Verification items for this drawing (mm, ordinates from the low corner). A direction names the side the tool comes from. Give positions to 0.01 mm unless a question says otherwise; leave off trailing zeros. Write each loop counter-clockwise with the first axis right and the second up, starting at its lowest first coordinate (ties: lowest second). Pieces come first, ordered by that corner, then holes. Notation, with made-up numbers: (84, 70.25) -> (97, 70.25) arc R20 cw to (97, 94.25) -> close; hole circle Ø7 at (13, 45). An arc over 180 degrees is marked (long way). Answer as a JSON object with one key per item and string values.
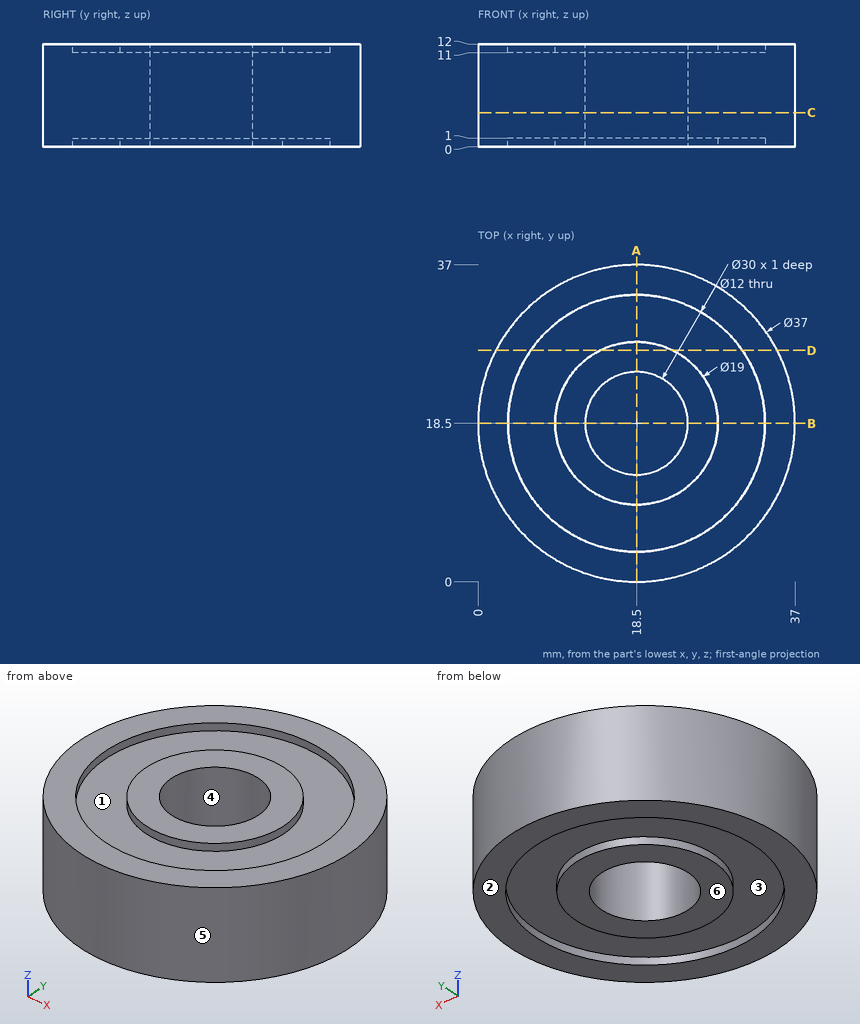
1. Scan lines: L1, parallel to Y at x = 18.5, z = 11.55; L2, parallel to Y at x = 18.5, z = 8; L3, parallel to Z at x = 4.5, y = 21. Record each from-to range of solid material in increasing order. Write a range as [from, to].
Determined:
{"L1": "[0, 3.5], [9, 12.5], [24.5, 28], [33.5, 37]", "L2": "[0, 12.5], [24.5, 37]", "L3": "[1, 11]"}
2. Mould release check, pull along X, two halves, no side actions. Record for the marked faces 4, 5 and 6: released by +X, released by -X, zero draft, split by the parting line, or undercut.
Determined:
{"face 4": "undercut", "face 5": "split by the parting line", "face 6": "zero draft"}
3. Sectioned sample at C-C, the plane z = 4. Enter the section's corners in (x, y), plus the area to 3 significant figures.
Determined:
{"outline": "circle Ø37 at (18.5, 18.5); hole circle Ø12 at (18.5, 18.5)", "area": "962 mm^2"}
4. Sectioned sample at D-D, the plane y = 27. Enter the section's corners in (x, z).
Determined:
{"outline": "(2.07, 0) -> (6.14, 0) -> (6.14, 1) -> (14.26, 1) -> (14.26, 0) -> (22.74, 0) -> (22.74, 1) -> (30.86, 1) -> (30.86, 0) -> (34.93, 0) -> (34.93, 12) -> (30.86, 12) -> (30.86, 11) -> (22.74, 11) -> (22.74, 12) -> (14.26, 12) -> (14.26, 11) -> (6.14, 11) -> (6.14, 12) -> (2.07, 12) -> close"}
5. Go/stop test with flat-tipped pins: P1, Ø5, axis at x = 22.5, z = 1.5, coming from the +Y side; P2, Ø1, axis at y = 4.5, z = 10, coming from the +X side; P3, Ø2, axis at x = 15.5, y = 5.5, coming from the -Z side; P4, Ø7, axis at x = 18.5, y = 18.5, coming from the +Z side. Record where each tip stops, or that it passes through.
Determined:
{"P1": "y = 36.94", "P2": "x = 31.15", "P3": "z = 1", "P4": "through"}
6. Sectioned sample at A-A, the plane x = 18.5. Enter the section's corners in (y, z), plus the area to 3 significant figures.
Determined:
{"outline": "(0, 0) -> (3.5, 0) -> (3.5, 1) -> (9, 1) -> (9, 0) -> (12.5, 0) -> (12.5, 12) -> (9, 12) -> (9, 11) -> (3.5, 11) -> (3.5, 12) -> (0, 12) -> close; (24.5, 0) -> (28, 0) -> (28, 1) -> (33.5, 1) -> (33.5, 0) -> (37, 0) -> (37, 12) -> (33.5, 12) -> (33.5, 11) -> (28, 11) -> (28, 12) -> (24.5, 12) -> close", "area": "278 mm^2"}
7. Access from +Z, -Z, +X, -X, +Y, -Y to the whole of each face (thin tool, end or side, straight path). Record for the marked faces 1, 2 and 3.
Determined:
{"face 1": "+Z", "face 2": "-Z, +X, -X, +Y, -Y", "face 3": "-Z"}
